```python
from build123d import *

# Parameters (mm, degrees)
F0_W      = 250
F0_H      = 20
F1_DEPTH  = 12.5
F2_R      = 7
F4_COUNT  = 5
F5_R      = 11
F6_DEPTH  = 300
F7_R      = 11
F8_DEPTH  = 50
F9_W      = 50
F9_H      = 450
F10_DEPTH = 580
F12_DEPTH = 25
F14_R     = 40
F15_R     = 10
F16_R     = 15


with BuildPart() as f1:
    # F0 (on Front) → F1 (new body, symmetric)
    with BuildSketch(Plane.XZ):
        with Locations((-125, 10)):
            Rectangle(F0_W, F0_H)
    extrude(amount=F1_DEPTH, both=True)

    # F2
    f2_edges = [f1.edges().sort_by_distance(p)[0] for p in [
        (-125, -12.5, 20),
        (-250, 0, 20),
        (-125, 12.5, 20),
    ]]
    fillet(f2_edges, radius=F2_R)

    # F4: F1 ×5 about axis
    f4_axis = Axis((0, 0, 61.4663511515), (0, 0, 1))


with BuildPart() as f1_1:
    add(f1.part)
    for i in range(1, F4_COUNT):
        add(f1.part.rotate(f4_axis, i * 360 / F4_COUNT))

    # F5 (on face) → F6 (join)
    with BuildSketch(Plane.XY.offset(20)):
        Circle(F5_R)
    extrude(amount=F6_DEPTH)

    # F7 (on face) → F8 (join)
    with BuildSketch(Plane.XY.offset(320)):
        with BuildLine():
            Line((270, -225), (270, 225))
            Line((270, 225), (-230, 225))
            ThreePointArc((-230, 225), (-258.2842712475, 213.2842712475), (-270, 185))
            Line((-270, 185), (-270, -185))
            ThreePointArc((-270, -185), (-258.2842712475, -213.2842712475), (-230, -225))
            Line((-230, -225), (270, -225))
        make_face()
        Circle(F7_R, mode=Mode.SUBTRACT)
        Circle(F7_R)
    extrude(amount=F8_DEPTH)

    # F9 (on face) → F10 (join)
    with BuildSketch(Plane.XY.offset(370)):
        with Locations((245, 0)):
            Rectangle(F9_W, F9_H)
    extrude(amount=F10_DEPTH)

    # F11 (on face) → F12 (join)
    with BuildSketch(Plane.XZ.offset(225)):
        with BuildLine():
            Line((220, 570), (220, 600))
            Line((220, 600), (-84.2436446853, 600))
            ThreePointArc((-84.2436446853, 600), (-109.3320234718, 586.4491109141), (-111.7557463729, 558.0382166576))
            Line((-111.7557463729, 558.0382166576), (-30, 370))
            Line((-30, 370), (-8.1914152974, 370))
            Line((-8.1914152974, 370), (-76.9036834094, 528.0382166576))
            ThreePointArc((-76.9036834094, 528.0382166576), (-74.4799605083, 556.4491109141), (-49.3915817218, 570))
            Line((-49.3915817218, 570), (220, 570))
        make_face()
    extrude(amount=-F12_DEPTH)

    # F13: F1 across plane


with BuildPart() as f1_2:
    add(f1_1.part)
    add(f1_1.part.mirror(Plane.XZ))

    # F14
    f14_edges = [f1_2.edges().sort_by_distance(p)[0] for p in [
        (245, -225, 950),
        (245, 225, 950),
    ]]
    fillet(f14_edges, radius=F14_R)

    # F15
    f15_edges = [f1_2.edges().sort_by_distance(p)[0] for p in [
        (220, 0, 950),
        (220, -213.284271, 938.284271),
        (220, -225, 755),
        (220, 225, 755),
        (220, 213.284271, 938.284271),
        (220, 225, 470),
        (220, -225, 470),
        (105.904292, -225, 370),
        (-130, -225, 370),
        (105.904292, 225, 370),
    ]]
    fillet(f15_edges, radius=F15_R)

    # F16
    f16_edges = [f1_2.edges().sort_by_distance(p)[0] for p in [
        (270, 0, 320),
    ]]
    fillet(f16_edges, radius=F16_R)


solid = f1_2.part
```
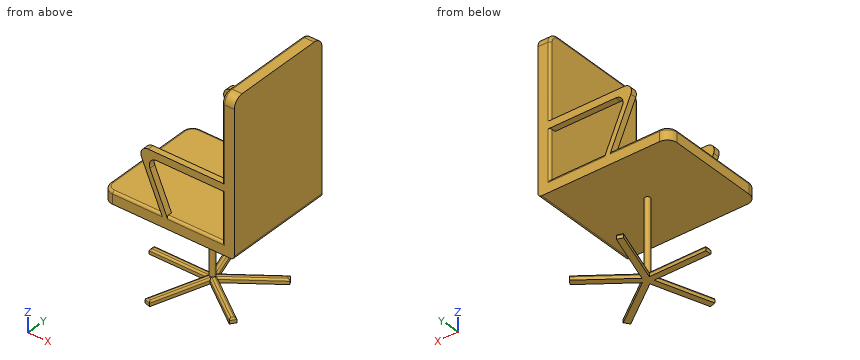
Part model, mm, in its own coordinate system. Round coordinates to 2 decimals unless told otherwise and drop trailing zeros. Order: outer loops, then holes, each group sorted by start corner. A loop starts at its lowest first (then second) coordinate and runs counter-clockwise, first axis right, second up. Notation, with made-up numbers: M -7,-19 L 32,-19 A17 ccw 32,5 Z; hole C 87.5,31.5 d6. An arc over 180 degrees is marked long. Put each result on its own line as item: value. Start each with the question number.
1. Slice it at B-B on z = 450. List the corners of the cut face in (x, y), then the cut area to 3 significant figures.
2. Slice it at D-D on z = 133. List the corners of the cut face in (x, y).
3. Drill centre lines: probe 1 along Z at (x, y) = (-44.5, 212); probe 2 along X at (y, z) = (86, 893.5); probe 3 along Z at (x, y) = (-226, 180). Where is each one in solid material? Low to high. Write a range as [from, to].
4. Slice it at A-A on x = -197. List the corners of the cut face in (y, z), then the cut area to 3 significant figures.
5. Slice it at C-C on y = 89.5. State how many separate pieces and enclosed holes the cut face has, then the cut area to 3 significant figures.
6. Drop flat-ended pins along their axis: pin 1 (6 mm diameter, centred on x = -189, y = -32, fed in from +Z); pin 2 (6.5 mm diameter, centred on x = -95, z = 5.5, fed in from +Y); pin 3 (20 mm diameter, centred on x = 113, y = -216, fed in from -Z). Give the stop position or say it passes through.
Findings:
1. outline: M -64.78,-225 L -42.97,-225 L -42.97,-200 L -64.78,-200 Z; M -64.78,200 L -42.97,200 L -42.97,225 L -64.78,225 Z; M 220,-215 A10 ccw 230,-225 L 270,-225 L 270,225 L 230,225 A10 ccw 220,215 Z
1. area: 23,500 mm2
2. outline: C 0,0 d22
3. probe 1: [320, 370], [403.35, 453.51], [570, 600]
3. probe 2: [220, 270]
3. probe 3: [320, 370]
4. outline: M -225,320 L 225,320 L 225,360 A10 ccw 215,370 L -215,370 A10 ccw -225,360 Z; M -12.5,0 L 12.5,0 L 12.5,13 A7 ccw 5.5,20 L -5.5,20 A7 ccw -12.5,13 Z
4. area: 22,900 mm2
5. separate pieces: 3
5. enclosed holes: 0
5. area: 57,200 mm2
6. pin 1: z = 370
6. pin 2: y = 12.5
6. pin 3: z = 320
